```python
from build123d import *

# Parameters (mm, degrees)
SKETCH2_R           = 3.75
BOSS_EXTRUDE1_DEPTH = 16
SKETCH3_R           = 3
CUT_EXTRUDE1_DEPTH  = 131
CUT_EXTRUDE2_DEPTH  = 31
CUT_EXTRUDE3_START  = -4
CUT_EXTRUDE3_DEPTH  = 30
CUT_EXTRUDE4_START  = -4
CUT_EXTRUDE4_DEPTH  = 30
FILLET1_R           = 6


with BuildPart() as part:
    # Sketch2 → Boss-Extrude1 (new body)
    with BuildSketch(Plane.XY):
        Polygon((-65, 0), (65, 0), (65, -30), (61, -30), (26.358983849, -10), (-26.358983849, -10), (-61, -30), (-65, -30), align=None)
        with Locations((-57, -8)):
            Circle(SKETCH2_R, mode=Mode.SUBTRACT)
        with Locations((57, -8)):
            Circle(SKETCH2_R, mode=Mode.SUBTRACT)
    extrude(amount=BOSS_EXTRUDE1_DEPTH)

    # Sketch3 → Cut-Extrude1 (cut, through all)
    with BuildSketch(Plane(origin=(65, 0, 0), x_dir=(0, 0, -1), z_dir=(1, 0, 0))):
        with Locations((-10, -23)):
            Circle(SKETCH3_R)
    extrude(amount=-CUT_EXTRUDE1_DEPTH, mode=Mode.SUBTRACT)

    # Sketch4 → Cut-Extrude2 (cut, through all)
    with BuildSketch(Plane(origin=(0, 0, 0), x_dir=(1, 0, 0), z_dir=(0, 1, 0))):
        Polygon((-51, -16), (-41, -6), (41, -6), (51, -16), align=None)
    extrude(amount=-CUT_EXTRUDE2_DEPTH, mode=Mode.SUBTRACT)

    # Sketch5 → Cut-Extrude3 (cut)
    with BuildSketch(Plane.ZY.offset(65).offset(CUT_EXTRUDE3_START)):
        with BuildLine():
            Line((4, -23), (4, -30))
            Line((4, -30), (16, -30))
            Line((16, -30), (16, -17))
            Line((16, -17), (10, -17))
            ThreePointArc((10, -17), (5.757359313, -18.757359313), (4, -23))
        make_face()
    extrude(amount=-CUT_EXTRUDE3_DEPTH, mode=Mode.SUBTRACT)

    # Sketch6 → Cut-Extrude4 (cut)
    with BuildSketch(Plane(origin=(65, 0, 0), x_dir=(0, 0, -1), z_dir=(1, 0, 0)).offset(CUT_EXTRUDE4_START)):
        with BuildLine():
            Line((-10, -17), (-16, -17))
            Line((-16, -17), (-16, -30))
            Line((-16, -30), (-4, -30))
            Line((-4, -30), (-4, -23))
            ThreePointArc((-4, -23), (-5.757359313, -18.757359313), (-10, -17))
        make_face()
    extrude(amount=-CUT_EXTRUDE4_DEPTH, mode=Mode.SUBTRACT)

    # Fillet1
    fillet1_edges = [part.edges().sort_by_distance(p)[0] for p in [
        (41, -9.226497308, 6),
        (-41, -9.226497308, 6),
        (-26.358983849, -10, 3),
        (26.358983849, -10, 3),
        (63, -30, 16),
        (-63, -30, 16),
    ]]
    fillet(fillet1_edges, radius=FILLET1_R)


solid = part.part
```
CAD build for the part. Positions are in the model's coordinates, mm. A direction names the side the tool comes from. Coordinates: 2 decimals unless noted, no trailing zeros. Loops run counter-clockwise (first coordinate to the right, second up) from the corner with the lowest first, then second, coordinate; pieces in that order, holes last. Notation, with made-up numbers: (70, 18.25) - (117, 18.25) arc R16 ccw to (117, 48.25) - close; hole circle Ø11 at (89, 65). An arc over 180 degrees is marked (long way). Return JSON: item names as keys, results as strings.
1. Band-saw the part on C-C (x = -57). Give the cut face in (y, z), and give its area (3 significant figures).
Result:
{"outline": "(-27.69, 0) - (-11.75, 0) - (-11.75, 16) - (-17, 16) - (-17, 10) arc R6 cw to (-23, 4) - (-27.69, 4) - close; (-4.25, 0) - (0, 0) - (0, 16) - (-4.25, 16) - close", "area": "202 mm2"}
2. Probe L1, parallel to Y at x = 63.15, z = 10; L2, parallel to X at y = -9.5, z = 2.75; L3, parallel to X at y = -20, z = 14.75. List the from-to ranges inside material, lowest first. Write a range as from..to.
Result:
{"L1": "y = -30..-26, -20..0", "L2": "x = -65..-60.44, -53.56..53.56, 60.44..65", "L3": "x = -65..-61, 61..65"}
3. 3-axis set-ups, long thin cutter, end or side, ignore diameter. For faces 1 (the cylindrical face through (-26.33, -10.21, 3.04)), 2 (the flat face through (-1, 0, 4)), 3 (the cylindrical face through (60.577, -6.874, 7.888)), 4 (the flat face through (47, -9, 12)), 5 (the flat face through (61, -26.3, 10.1)): which of +Z, -Z, +X, -X, +Y, -Y reach the whole face in a straight line?
Result:
{"face 1": "+Z, -Z, -Y", "face 2": "+Z, -Z, +X, -X, +Y", "face 3": "+Z, -Z", "face 4": "+Z, +Y, -Y", "face 5": "+Z, -Y"}
4. Band-saw the part on D-D (y = -27.5). Give the cut face in (x, z).
Result:
{"outline": "(-65, 0) - (-56.67, 0) - (-56.67, 4) - (-61, 4) - (-61, 14.87) - (-65, 14.87) - close; (56.67, 0) - (65, 0) - (65, 14.87) - (61, 14.87) - (61, 4) - (56.67, 4) - close"}
5. Band-saw the part on A-A (y = -8). Give the cut face in (x, z), and give its area (3 significant figures).
Result:
{"outline": "(-65, 0) - (-60.75, 0) - (-60.75, 16) - (-65, 16) - close; (-53.25, 0) - (53.25, 0) - (53.25, 16) - (51, 16) - (42.76, 7.76) arc R6 cw to (38.51, 6) - (-38.51, 6) arc R6 cw to (-42.76, 7.76) - (-51, 16) - (-53.25, 16) - close; (60.75, 0) - (65, 0) - (65, 16) - (60.75, 16) - close", "area": "922 mm2"}
6. Mould opens along Z. For faces 6 (the flat face through (-47, -9, 12)), 7 (the flat face through (55, -17, 13)), 8 (the cylindrical face through (63, -24.8, 12.4)) say: released by +Z, released by -Z, zero draft, split by the parting line, or undercut.
Result:
{"face 6": "released by +Z", "face 7": "zero draft", "face 8": "undercut"}
7. Drop flat-ended pins along their axis: pin 1 (7 mm diameter, centred on y = -23, z = 10, fed in from -X); pin 2 (5 mm diameter, centred on x = -2.5, z = 1.5, fed in from -Y); pin 3 (2 mm diameter, centred on x = -53, y = -25, fed in from +Z); pin 4 (1.8 mm diameter, centred on x = -52.5, z = 11.5, fed in from -Y). Give the stop position or say it passes through.
Result:
{"pin 1": "stops at x = -65", "pin 2": "stops at y = -10", "pin 3": "stops at z = 4", "pin 4": "stops at y = -17"}
8. Band-saw the part on B-B (z = 14.25). Give the cut face in (x, y).
Result:
{"outline": "(-65, -28.24) - (-61, -28.24) - (-61, -17) - (-49.25, -17) - (-49.25, 0) - (-65, 0) - close; (49.25, -17) - (61, -17) - (61, -28.24) - (65, -28.24) - (65, 0) - (49.25, 0) - close; hole circle Ø7.5 at (-57, -8); hole circle Ø7.5 at (57, -8)"}
